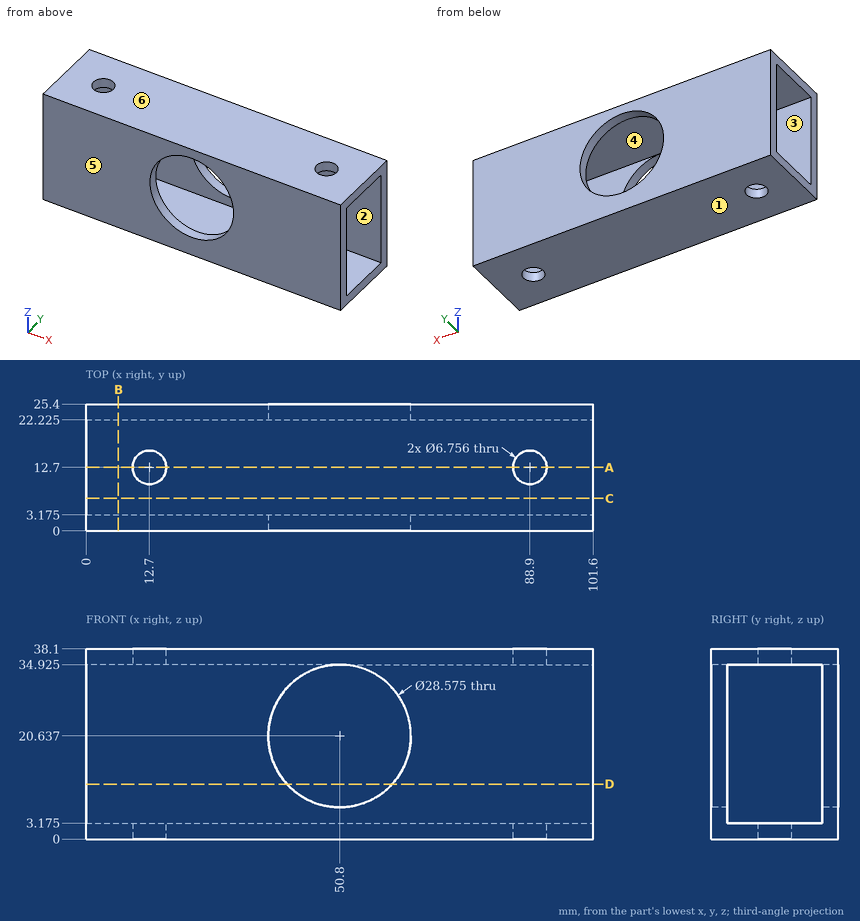
Can you work these out from the drawing? Everything is in mm from the part's minimum corner. A direction names the side the tool comes from. Give positions to 0.01 mm unless a question says otherwise; leave off trailing zeros. Order: outer loops, then holes, each group sorted by start corner. A loop starts at its lowest first (then second) coordinate and runs counter-clockwise, first axis right, second up. Notation, with made-up numbers: M 74.5,55 L 83.5,55 A33 cw 83.5,92 Z; hole C 88,-29.5 d7. An arc over 180 degrees is marked long. One line per item, written item: value.
Item 1: If we section it at D-D on z = 11: Write out the boundary of the cut face in (x, y) (1 decimal).
Verdict:
outline: M 0,0 L 40.3,0 L 40.3,3.2 L 0,3.2 Z; M 0,22.2 L 40.3,22.2 L 40.3,25.4 L 0,25.4 Z; M 61.3,0 L 101.6,0 L 101.6,3.2 L 61.3,3.2 Z; M 61.3,22.2 L 101.6,22.2 L 101.6,25.4 L 61.3,25.4 Z
Item 2: For the marked faces 1 and 2, which set-ups out of +Z, -Z, +X, -X, +Y, -Y let a thin tool reach every point of the face, with its end or its side?
Verdict:
face 1: -Z, +X, -X, +Y, -Y
face 2: +X, -X
Item 3: If we section it at A-A on y = 12.7: Write out the boundary of the cut face in (x, z) (1 decimal).
Verdict:
outline: M 0,0 L 9.3,0 L 9.3,3.2 L 0,3.2 Z; M 0,34.9 L 9.3,34.9 L 9.3,38.1 L 0,38.1 Z; M 16.1,0 L 85.5,0 L 85.5,3.2 L 16.1,3.2 Z; M 16.1,34.9 L 85.5,34.9 L 85.5,38.1 L 16.1,38.1 Z; M 92.3,0 L 101.6,0 L 101.6,3.2 L 92.3,3.2 Z; M 92.3,34.9 L 101.6,34.9 L 101.6,38.1 L 92.3,38.1 Z
Item 4: Please list where these lines run through material, in increasing order: line 1 (X direction, y = 12.7, z = 1.05); line 2 (Z direction, x = 53, y = 8.75) (1 decimal); line 3 (Y direction, x = 41.5, z = 33.5) (1 decimal).
Verdict:
line 1: 0 to 9.32, 16.08 to 85.52, 92.28 to 101.6
line 2: 0 to 3.2, 34.9 to 38.1
line 3: 0 to 3.2, 22.2 to 25.4
Item 5: If we section it at C-C on y = 6.5: Write out the boundary of the cut face in (x, z) (1 decimal).
Verdict:
outline: M 0,0 L 101.6,0 L 101.6,3.2 L 0,3.2 Z; M 0,34.9 L 101.6,34.9 L 101.6,38.1 L 0,38.1 Z
Item 6: If we mould it in two halves opening along Y, with no side actions, what happens to the marked faces 3, 4, 5 and 6? For each: pulls with the +Y half, pulls with the -Y half, needs draft (parallel to the pull), parting line crosses it, or undercut.
Verdict:
face 3: undercut
face 4: undercut
face 5: pulls with the -Y half
face 6: needs draft
Item 7: If we section it at B-B on x = 6.5: Write out the boundary of the cut face in (y, z) (1 decimal), and give its area (3 significant figures).
Verdict:
outline: M 0,0 L 25.4,0 L 25.4,38.1 L 0,38.1 Z; hole M 3.2,3.2 L 22.2,3.2 L 22.2,34.9 L 3.2,34.9 Z
area: 363 mm2
